Geometry check sheet. Reference: the model listing, model coordinates, mm. A direction names the side the tool comes from. Coordinates: 2 decimals unless noted, no trailing zeros. Loops run counter-clockwise (first coordinate to the right, second up) from the corner with the lowest first, then second, coordinate; pieces in that order, holes last.
from build123d import *

# Parameters (mm, degrees)
F0_W     = 42
F0_H     = 7
F1_DEPTH = 9
F0_R     = 7.5
F2_DEPTH = 30
F4_DEPTH = 18.5
F5_DEPTH = 11.5


with BuildPart() as f1:
    # F0 (on Top) → F1 (new body)
    with BuildSketch(Plane.XY):
        Polygon((-18.315635, 11.012554), (-18.315635, -0.487446), (14.684365, -0.487446), (23.684365, 8.512554), (23.684365, 11.012554), align=None)
        Polygon((14.684365, 29.512554), (-18.315635, 29.512554), (-18.315635, 18.012554), (23.684365, 18.012554), (23.684365, 20.512554), align=None)
        with Locations((2.684365, 14.512554)):
            Rectangle(F0_W, F0_H)
    extrude(amount=F1_DEPTH)

    # F0 (on Top) → F2 (join)
    with BuildSketch(Plane.XY):
        with BuildLine():
            Line((-18.315635, 29.512554), (-36.315635, 29.512554))
            ThreePointArc((-36.315635, 29.512554), (-51.315635, 14.512554), (-36.315635, -0.487446))
            Line((-36.315635, -0.487446), (-18.315635, -0.487446))
            Line((-18.315635, -0.487446), (-18.315635, 11.012554))
            Line((-18.315635, 11.012554), (-18.315635, 18.012554))
            Line((-18.315635, 18.012554), (-18.315635, 29.512554))
        make_face()
        with Locations((-36.315635, 14.512554)):
            Circle(F0_R, mode=Mode.SUBTRACT)
    extrude(amount=F2_DEPTH)

    # F3 (on Front) → F4 (join)
    with BuildSketch(Plane.XZ):
        Polygon((23.775358, 9.021481), (-18.101137, 29.923748), (-18.101137, 8.923748), align=None)
    extrude(amount=-F4_DEPTH)

    # F4_face (on face) → F5 (cut)
    with BuildSketch(Plane(origin=(-4.133589, 0, 15.976161), x_dir=(1, 0, 0), z_dir=(0, -1, 0))):
        Polygon((18.704939, -6.976161), (27.908947, -6.95468), (-13.967548, 13.947587), (-13.967548, -6.976161), align=None)
    extrude(amount=-F5_DEPTH, mode=Mode.SUBTRACT)


solid = f1.part
(1) Scan lines: L1, parallel to X at y = 12.75, z = 12.75; L2, parallel to Z at x = -7, y = 8; L3, parallel to X at y = 12.5, z = 15.25. Record each from-to range of solid material in increasing order.
Findings:
L1: x = -51.21 to -43.61, -29.03 to -18.32, -18.1 to 16.31
L2: z = 0 to 9
L3: x = -51.18 to -43.54, -29.09 to -18.32, -18.1 to 11.3
(2) Sectioned sample at A-A on z = 26. Record the cut outline in (x, y), and give its area (3 significant figures).
Findings:
outline: (-36.32, -0.49) - (-18.32, -0.49) - (-18.32, 29.51) - (-36.32, 29.51) arc R15 ccw to start; (-18.1, 11.5) - (-10.24, 11.5) - (-10.24, 18.5) - (-18.1, 18.5) - close; hole circle Ø15 at (-36.32, 14.51)
area: 772 mm2
(3) Sectioned sample at C-C on y = 12.5. Record the cut outline in (x, z).
Findings:
outline: (-51.18, 0) - (-43.54, 0) - (-43.54, 30) - (-51.18, 30) - close; (-29.09, 0) - (23.68, 0) - (23.68, 9) - (14.57, 9) - (23.78, 9.02) - (-18.1, 29.92) - (-18.1, 9) - (-18.32, 9) - (-18.32, 30) - (-29.09, 30) - close
(4) Gauge pin test, flat ends, axial feed: pin 1 Ø5.5 at (y, z) = (13.5, 18.5) entering from -X; pin 2 Ø4.5 at (y, z) = (15, 4) entering from +X; pin 3 Ø2 at (x, z) = (-1.5, 14) entering from -Y; pin 4 Ø3 at (y, z) = (3.5, 8) entering from +X. Record the tip position at first contact, or that the pin passes through.
Findings:
pin 1: stops at x = -51.32
pin 2: stops at x = 23.68
pin 3: stops at y = 11.5
pin 4: stops at x = 20.17
(5) Draft check along X on faces 1 (the flat face through (-28, 15, 30)), 2 (the flat face through (3.13, 14.951, 19.326)), 3 (the flat face through (-18.316, 14, 19)). Enter one of: +X half, -X half, draft (parallel to the pull), parting line (faces both ways), or undercut.
Findings:
face 1: draft
face 2: +X half
face 3: undercut
(6) Sectioned sample at B-B on x = 18.5. Record the cut outline in (y, z).
Findings:
outline: (3.33, 0) - (25.7, 0) - (25.7, 9) - (3.33, 9) - close; (11.5, 9.01) - (18.5, 9.01) - (18.5, 11.65) - (11.5, 11.65) - close
(7) Sectioned sample at D-D on z = 15.75. Record the cut outline in (x, y), and give its area (3 significant figures).
Findings:
outline: (-36.32, -0.49) - (-18.32, -0.49) - (-18.32, 29.51) - (-36.32, 29.51) arc R15 ccw to start; (-18.1, 11.5) - (10.3, 11.5) - (10.3, 18.5) - (-18.1, 18.5) - close; hole circle Ø15 at (-36.32, 14.51)
area: 915 mm2
(8) Access from +Z, -Z, +X, -X, +Y, -Y to the whole of each face (thin tool, end or side, straight path). Record for faces 4 (the flat face through (-2, 11.5, 17)), 5 (the flat face through (-18.101, 15, 20)), 6 (the flat face through (23.684, 14, 4)).
Findings:
face 4: +Z, +X, -Y
face 5: +Z, +Y, -Y
face 6: -Z, +X, +Y, -Y
